from build123d import *

# Parameters (mm, degrees)
SKETCH_1_W          = 42.5
SKETCH_1_H          = 42.5
SKETCH_1_R          = 2.025
SKETCH_1_R_2        = 18.5
EXTRUDE_1_DEPTH     = 5
EXTRUDE_START       = 5
SKETCH_1_3_W        = 42.5
SKETCH_1_3_H        = 42.5
SKETCH_1_3_R        = 2.025
SKETCH_1_3_R_2      = 18.5
SKETCH_1_3_R_3      = 5.515
EXTRUDE_2_DEPTH     = 3
CUT_EXTRUDE_1_DEPTH = 5
SKETCH_3_R          = 8
SKETCH_3_R_2        = 3.5
EXTRUDE_3_DEPTH     = 2


with BuildPart() as part:
    # 草图1 → 凸台-拉伸1 (new body)
    with BuildSketch(Plane(origin=(0, 0, 0), x_dir=(1, 0, 0), z_dir=(0, 1, 0))):
        Rectangle(SKETCH_1_W, SKETCH_1_H)
        with Locations(Location((-17.67766953, -17.67766953, 0), (0, 0, 270))):
            Circle(SKETCH_1_R, mode=Mode.SUBTRACT)
        with Locations(Location((17.67766953, -17.67766953, 0), (0, 0, 270))):
            Circle(SKETCH_1_R, mode=Mode.SUBTRACT)
        with Locations(Location((17.67766953, 17.67766953, 0), (0, 0, 270))):
            Circle(SKETCH_1_R, mode=Mode.SUBTRACT)
        with Locations(Location((-17.67766953, 17.67766953, 0), (0, 0, 270))):
            Circle(SKETCH_1_R, mode=Mode.SUBTRACT)
        with Locations(Location((0, 0, 0), (0, 0, 270))):
            Circle(SKETCH_1_R_2, mode=Mode.SUBTRACT)
    extrude(amount=EXTRUDE_1_DEPTH)

    # 草图1<3> → 凸台-拉伸2 (add)
    # profile 1 of 2: a face of its own
    with BuildSketch(Plane(origin=(0, 0, 0), x_dir=(1, 0, 0), z_dir=(0, 1, 0)).offset(EXTRUDE_START)):
        Rectangle(SKETCH_1_3_W, SKETCH_1_3_H)
        with Locations(Location((-17.67766953, -17.67766953, 0), (0, 0, 270))):
            Circle(SKETCH_1_3_R, mode=Mode.SUBTRACT)
        with Locations(Location((17.67766953, -17.67766953, 0), (0, 0, 270))):
            Circle(SKETCH_1_3_R, mode=Mode.SUBTRACT)
        with Locations(Location((17.67766953, 17.67766953, 0), (0, 0, 270))):
            Circle(SKETCH_1_3_R, mode=Mode.SUBTRACT)
        with Locations(Location((-17.67766953, 17.67766953, 0), (0, 0, 270))):
            Circle(SKETCH_1_3_R, mode=Mode.SUBTRACT)
        with Locations(Location((0, 0, 0), (0, 0, 270))):
            Circle(SKETCH_1_3_R_2, mode=Mode.SUBTRACT)
    # profile 2 of 2: a face of its own
    with BuildSketch(Plane(origin=(0, 0, 0), x_dir=(1, 0, 0), z_dir=(0, 1, 0)).offset(EXTRUDE_START)):
        with Locations(Location((0, 0, 0), (0, 0, 270))):
            Circle(SKETCH_1_3_R_2)
        with Locations(Location((0, 0, 0), (0, 0, 270))):
            Circle(SKETCH_1_3_R_3, mode=Mode.SUBTRACT)
    extrude(amount=EXTRUDE_2_DEPTH)

    # 草图2 → 切除-拉伸1 (cut)
    with BuildSketch(Plane(origin=(0, 8, 0), x_dir=(1, 0, 0), z_dir=(0, 1, 0))):
        with BuildLine():
            Line((-17.67766953, -12.67766953), (-21.25, -12.67766953))
            Line((-21.25, -12.67766953), (-21.25, -21.25))
            Line((-21.25, -21.25), (-12.67766953, -21.25))
            Line((-12.67766953, -21.25), (-12.67766953, -17.67766953))
            ThreePointArc((-12.67766953, -17.67766953), (-14.142135624, -14.142135624), (-17.67766953, -12.67766953))
        make_face()
        with BuildLine():
            Line((21.25, 21.25), (12.67766953, 21.25))
            Line((12.67766953, 21.25), (12.67766953, 17.67766953))
            ThreePointArc((12.67766953, 17.67766953), (14.142135624, 14.142135624), (17.67766953, 12.67766953))
            Line((17.67766953, 12.67766953), (21.25, 12.67766953))
            Line((21.25, 12.67766953), (21.25, 21.25))
        make_face()
    extrude(amount=-CUT_EXTRUDE_1_DEPTH, mode=Mode.SUBTRACT)

    # 草图3 → 凸台-拉伸3 (add)
    with BuildSketch(Plane(origin=(0, 8, 0), x_dir=(1, 0, 0), z_dir=(0, 1, 0))):
        with Locations(Location((0, 0, 0), (0, 0, 90))):
            Circle(SKETCH_3_R)
        with Locations(Location((0, 0, 0), (0, 0, 270))):
            Circle(SKETCH_3_R_2, mode=Mode.SUBTRACT)
    extrude(amount=EXTRUDE_3_DEPTH)


solid = part.part
Geometry: final body of the model. Coordinates: model frame, mm. A direction names the side the tool comes from. Round coordinates to 2 decimals unless told otherwise and drop trailing zeros. Loops run counter-clockwise (first coordinate to the right, second up) from the corner with the lowest first, then second, coordinate; pieces in that order, holes last. Notation, with made-up numbers: (-20, 12) -> (14, 12) arc R21 ccw to (14, 39) -> close; hole circle Ø5 at (1, -30.75). An arc over 180 degrees is marked (long way). One line per question, with ' | ' between items. Start each with the question number.
1. Section D-D on x = 5. Output: boundary loops of the cut face in (y, z) (3 decimals).
2. Section B-B on x = 0. Output: boundary loops of the cut face in (y, z) (3 decimals), and give its area (3 significant figures).
3. Set-up query: faces 1 (the face through (-17.069, 3.944, -15.746)), 2 (the face through (-19, 6, 12.678)), 3 (the face through (16, 3, -16)), 4 (the face through (4.4, 5, 3.9)), 5 (the face through (7.81, 8.99, 1.73)). Return all of +Z, -Z, +X, -X, +Y, -Y with unobstructed straight access to the full face (end or side cutting, diameter ignored); none if empty.
4. Line query: line 1 along X through (y, z) = (6.5, 0) (3 decimals); line 2 along X through (y, z) = (9.3, 0); line 3 along Y through (x, z) = (-16.5, 7.5). Output: solid intervals per line, ascending. Write a range as [from, to].
5. Contact query for flat-ended pins moving along their axis: pin 1 (8 mm diameter, centred on x = 0, z = 0, fed in from -Y); pin 2 (4 mm diameter, centred on x = 7, z = -3.5, fed in from -Y); pin 3 (4 mm diameter, centred on x = 15.5, y = 9, fed in from -Z). Output: stop coordinate, or through.
6. Mould query, pull axis X, two halves, no side actions, for faces 6 (the face through (5.468, 6.479, -0.718)), 7 (the face through (-10, 8, 0)), 8 (the face through (14.103, 5.535, -14.181)). Classes: pulls with the +X half, pulls with the -X half, needs draft (parallel to the pull), parting line crosses it, or undercut.
7. Section C-C on z = 0. Output: boundary loops of the cut face in (x, y) (3 decimals), and give its area (3 significant figures).
8. Section A-A on y = 7. Output: boundary loops of the cut face in (x, z) (3 decimals).
Returned:
1) outline: (0, -21.25) -> (8, -21.25) -> (8, -6.245) -> (10, -6.245) -> (10, 6.245) -> (8, 6.245) -> (8, 21.25) -> (0, 21.25) -> (0, 17.812) -> (5, 17.812) -> (5, 2.327) -> (8, 2.327) -> (8, -2.327) -> (5, -2.327) -> (5, -17.812) -> (0, -17.812) -> close
2) outline: (0, -21.25) -> (8, -21.25) -> (8, -8) -> (10, -8) -> (10, -3.5) -> (8, -3.5) -> (8, -5.515) -> (5, -5.515) -> (5, -18.5) -> (0, -18.5) -> close; (0, 18.5) -> (5, 18.5) -> (5, 5.515) -> (8, 5.515) -> (8, 3.5) -> (10, 3.5) -> (10, 8) -> (8, 8) -> (8, 21.25) -> (0, 21.25) -> close | area: 140 mm2
3) face 1: +Y, -Y | face 2: +Z, -X, +Y | face 3: -Z, +X, +Y | face 4: -Y | face 5: +Y
4) line 1: x = [-21.25, -5.515], [5.515, 21.25] | line 2: x = [-8, -3.5], [3.5, 8] | line 3: y = [5, 8]
5) pin 1: stops at y = 8 | pin 2: stops at y = 5 | pin 3: stops at z = -14.56
6) face 6: undercut | face 7: needs draft | face 8: pulls with the +X half
7) outline: (-21.25, 0) -> (-18.5, 0) -> (-18.5, 5) -> (-5.515, 5) -> (-5.515, 8) -> (-3.5, 8) -> (-3.5, 10) -> (-8, 10) -> (-8, 8) -> (-21.25, 8) -> close; (3.5, 8) -> (5.515, 8) -> (5.515, 5) -> (18.5, 5) -> (18.5, 0) -> (21.25, 0) -> (21.25, 8) -> (8, 8) -> (8, 10) -> (3.5, 10) -> close | area: 140 mm2
8) outline: (-21.25, -21.25) -> (12.678, -21.25) -> (12.678, -17.678) arc R5 cw to (17.678, -12.678) -> (21.25, -12.678) -> (21.25, 21.25) -> (-12.678, 21.25) -> (-12.678, 17.678) arc R5 cw to (-17.678, 12.678) -> (-21.25, 12.678) -> close; hole circle Ø4.05 at (-17.678, -17.678); hole circle Ø11.03 at (0, 0); hole circle Ø4.05 at (17.678, 17.678)
